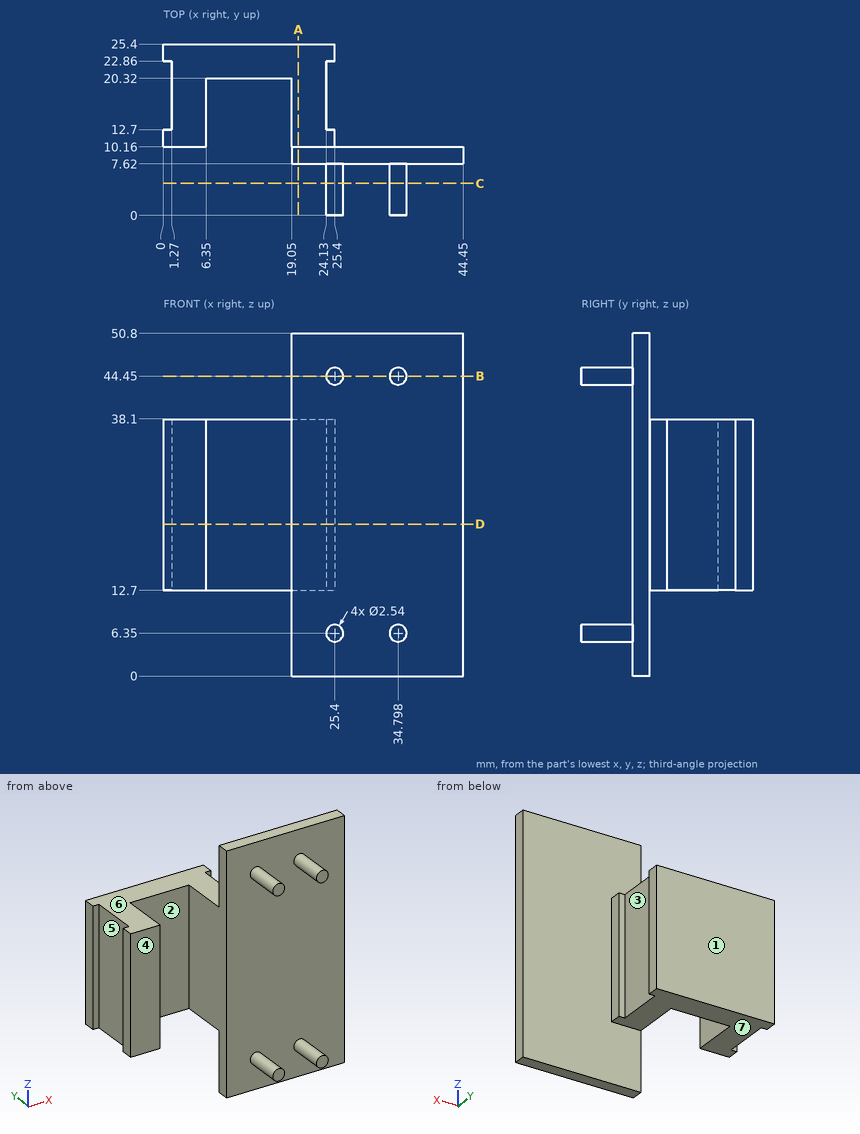
For this review, use the dimensioned drawing (mm, ordinates from the lowest corner) and the shaded views. A direction names the side the tool comes from. Round coordinates to 2 decimals unless told otherwise and drop trailing zeros. Write each loop counter-clockwise with the first axis right and the second up, starting at its lowest first coordinate (ties: lowest second). Pieces come first, ordered by that corner, then holes. Notation, with made-up numbers: (14.5, 31.5) - (58.5, 31.5) arc R27 cw to (58.5, 61.5) - close; hole circle Ø5 at (27, 84). An arc over 180 degrees is marked (long way). One line per item, written item: value. Start each with the question number.
1. Clearance check with flat-ended pins moving along their axes: P1, Ø3, axis at y = 12.5, z = 23, coming from the +X side; P2, Ø5, axis at y = 17, z = 24.5, coming from the -X side; P3, Ø1, axis at x = 36, z = 23.5, coming from the +Y side; P4, Ø4, axis at y = 5, z = 29.5, coming from the -X side. State where each tip first meets the part, or that it passes through.
2. Consider section D-D on z = 22.5. Write out the cut boundary in (x, y), and give its area (3 significant figures).
3. The part is to be moulded in two halves that separate along X. For the marked faces 1, 2 and 3, say which applies: released by +X, released by -X, zero draft, split by the parting line, or undercut.
4. Machinability: for the marked faces 4, 5, 6 and 7, which of the approach directions +Z, -Z, +X, -X, +Y, -Y give a long, thin tool a straight path to every point of the face, cutting with its end or side? Answer none if there is none.
5. Consider section C-C on y = 4.75. Write out the cut boundary in (x, z), and give its area (3 significant figures).
6. To check wall thickness, follow L1, parallel to X at y = 14.75, z = 25; L2, parallel to Y at x = 42, z = 3; L3, parallel to Z at x = 24, y = 10.5. State the ranges of each line that lie inside material, in increasing order. Write a range as from..to.
7. Consider section A-A on x = 20. Write out the cut boundary in (y, z), and give its area (3 significant figures).
8. Consider section B-B on z = 44.45. Write out the cut boundary in (x, y), and give its area (3 significant figures).
Checks:
1. P1: stops at x = 25.4
1. P2: stops at x = 1.27
1. P3: stops at y = 10.16
1. P4: passes through
2. outline: (0, 10.16) - (6.35, 10.16) - (6.35, 20.32) - (19.05, 20.32) - (19.05, 7.62) - (44.45, 7.62) - (44.45, 10.16) - (25.4, 10.16) - (25.4, 12.7) - (24.13, 12.7) - (24.13, 22.86) - (25.4, 22.86) - (25.4, 25.4) - (0, 25.4) - (0, 22.86) - (1.27, 22.86) - (1.27, 12.7) - (0, 12.7) - close
2. area: 297 mm^2
3. face 1: zero draft
3. face 2: undercut
3. face 3: released by +X
4. face 4: +Z, -Z, -X, -Y
4. face 5: +Z, -Z, -X
4. face 6: +Z, +X, -X, +Y
4. face 7: -Z, +X, -X, +Y
5. outline: circle Ø2.54 at (25.4, 6.35); circle Ø2.54 at (25.4, 44.45); circle Ø2.54 at (34.8, 6.35); circle Ø2.54 at (34.8, 44.45)
5. area: 20.3 mm^2
6. L1: x = 1.27..6.35, 19.05..24.13
6. L2: y = 7.62..10.16
6. L3: z = 12.7..38.1
7. outline: (7.62, 0) - (10.16, 0) - (10.16, 12.7) - (25.4, 12.7) - (25.4, 38.1) - (10.16, 38.1) - (10.16, 50.8) - (7.62, 50.8) - close
7. area: 516 mm^2
8. outline: (19.05, 7.62) - (24.13, 7.62) - (24.13, 0) - (26.67, 0) - (26.67, 7.62) - (33.53, 7.62) - (33.53, 0) - (36.07, 0) - (36.07, 7.62) - (44.45, 7.62) - (44.45, 10.16) - (19.05, 10.16) - close
8. area: 103 mm^2
